Build history of the part. All positions in model axes, mm. A direction names the side the tool comes from. Coordinates: 2 decimals unless noted, no trailing zeros. Order: outer loops, then holes, each group sorted by start corner. A loop starts at its lowest first (then second) coordinate and runs counter-clockwise, first axis right, second up. Notation, with made-up numbers: (37.5, 85.5) - (63.5, 85.5) arc R35 ccw to (63.5, 117.5) - close; hole circle Ø7 at (66.25, 57). An arc over 180 degrees is marked (long way). Return JSON: item names as keys, results as strings.
from build123d import *

# Parameters (mm, degrees)
EXTRUDE_1_DEPTH     = 45
SKETCH_2_R          = 2.4
CUT_EXTRUDE_1_DEPTH = 9


with BuildPart() as part:
    # Sketch 1 → Extrude 1 (new body)
    with BuildSketch(Plane(origin=(0, 0, 0), x_dir=(0, 0, -1), z_dir=(1, 0, 0))):
        with BuildLine():
            Line((-22.5, 20), (22.5, 20))
            Line((22.5, 20), (22.5, -13))
            Line((22.5, -13), (10.908295205, -13))
            Line((10.908295205, -13), (5.142300877, -6.128355545))
            ThreePointArc((5.142300877, -6.128355545), (0, 8), (-5.142300877, -6.128355545))
            Line((-5.142300877, -6.128355545), (-10.908295205, -13))
            Line((-10.908295205, -13), (-22.5, -13))
            Line((-22.5, -13), (-22.5, 20))
        make_face()
    extrude(amount=EXTRUDE_1_DEPTH)

    # Sketch 2 → Cut-Extrude 1 (cut)
    with BuildSketch(Plane(origin=(0, 20, 0), x_dir=(1, 0, 0), z_dir=(0, 1, 0))):
        with Locations(Location((7.5, 16, 0), (0, 0, 270))):
            Circle(SKETCH_2_R)
        with Locations(Location((37.5, 16, 0), (0, 0, 270))):
            Circle(SKETCH_2_R)
        with Locations(Location((37.5, -16, 0), (0, 0, 270))):
            Circle(SKETCH_2_R)
        with Locations(Location((7.5, -16, 0), (0, 0, 270))):
            Circle(SKETCH_2_R)
    extrude(amount=-CUT_EXTRUDE_1_DEPTH, mode=Mode.SUBTRACT)


solid = part.part
1. Cut at B-B on x = 41. Give the cut face in (y, z).
Check values:
{"outline": "(-13, -22.5) - (20, -22.5) - (20, 22.5) - (-13, 22.5) - (-13, 10.91) - (-6.13, 5.14) arc R8 cw (long way) to (-6.13, -5.14) - (-13, -10.91) - close"}
2. Drop flat-ended pins along their axis: pin 1 (2.5 mm diameter, centred on x = 8, z = 16, fed in from +Y); pin 2 (14.5 mm diameter, centred on y = 0, z = 0, fed in from -X). Give the stop position or say it passes through.
Check values:
{"pin 1": "y = 11", "pin 2": "through"}
3. Cut at A-A on y = 0. Give the cut face in (x, z), plus the area to 4 significant figures.
Check values:
{"outline": "(0, -22.5) - (45, -22.5) - (45, -8) - (0, -8) - close; (0, 8) - (45, 8) - (45, 22.5) - (0, 22.5) - close", "area": "1,305 mm²"}
4. Cut at D-D on z = 6.5. Give the cut face in (x, y), plus the area to 3 significant figures.
Check values:
{"outline": "(0, -7.75) - (45, -7.75) - (45, -4.66) - (0, -4.66) - close; (0, 4.66) - (45, 4.66) - (45, 20) - (0, 20) - close", "area": "829 mm²"}
5. Probe L1, parallel to X at y = 17, z = -16; L2, parallel to Z at x = 37, y = 17; L3, parallel to Z at x = 9.5, y = 13.5. List the from-to ranges inside material, lowest first.
Check values:
{"L1": "0 to 5.1, 9.9 to 35.1, 39.9 to 45", "L2": "-22.5 to -18.35, -13.65 to 13.65, 18.35 to 22.5", "L3": "-22.5 to -17.33, -14.67 to 14.67, 17.33 to 22.5"}
6. Mould opens along Z. For faces 4 (the flat face through (8, 11, -16)), 5 (the flat face through (22, 3, 22.5)), 6 (the flat face through (22, -13, 17)) say: pulls with the +Z half, pulls with the -Z half, needs draft (parallel to the pull), parting line crosses it, or undercut.
Check values:
{"face 4": "undercut", "face 5": "pulls with the +Z half", "face 6": "needs draft"}
7. Cut at C-C on z = 16. Give the cut face in (x, y), plus the area to 3 significant figures.
Check values:
{"outline": "(0, -13) - (45, -13) - (45, 20) - (39.9, 20) - (39.9, 11) - (35.1, 11) - (35.1, 20) - (9.9, 20) - (9.9, 11) - (5.1, 11) - (5.1, 20) - (0, 20) - close", "area": "1,400 mm²"}
8. Tool access for faces 1 (the flat face through (22, 4, -22.5)), 2 (the flat face through (22.185, -9.516, 7.985)), 3 (the flat face through (38, 11, 16)): list every direction of +Z, -Z, +X, -X, +Y, -Y with a clear straight run to the whole face (end or side of a thin tool).
Check values:
{"face 1": "-Z, +X, -X, +Y, -Y", "face 2": "+X, -X, -Y", "face 3": "+Y"}
